```python
from build123d import *

# Parameters (mm, degrees)
SKETCH9_R           = 13.427276503
SKETCH9_R_2         = 5
BOSS_EXTRUDE1_DEPTH = 1
FILLET1_R           = 6
BOSS_EXTRUDE2_START = -3
SKETCH14_R          = 5
BOSS_EXTRUDE2_DEPTH = 5
BOSS_EXTRUDE3_START = -2
SKETCH15_R          = 6
BOSS_EXTRUDE3_DEPTH = 3
CIRPATTERN1_COUNT   = 3


with BuildPart() as part:
    # Sketch9 → Boss-Extrude1 (new body)
    with BuildSketch(Plane.XY):
        with BuildLine():
            Line((-11, 30.049958403), (-11, 21.330729008))
            ThreePointArc((-11, 21.330729008), (-20.784609691, 12), (-23.972953202, -1.139085062))
            Line((-23.972953202, -1.139085062), (-31.524027359, -5.49869976))
            ThreePointArc((-31.524027359, -5.49869976), (-27.712812921, -16), (-20.524027359, -24.551258643))
            Line((-20.524027359, -24.551258643), (-12.972953202, -20.191643945))
            ThreePointArc((-12.972953202, -20.191643945), (0, -24), (12.972953202, -20.191643945))
            Line((12.972953202, -20.191643945), (20.524027359, -24.551258643))
            ThreePointArc((20.524027359, -24.551258643), (27.712812921, -16), (31.524027359, -5.49869976))
            Line((31.524027359, -5.49869976), (23.972953202, -1.139085062))
            ThreePointArc((23.972953202, -1.139085062), (20.784609691, 12), (11, 21.330729008))
            Line((11, 21.330729008), (11, 30.049958403))
            ThreePointArc((11, 30.049958403), (0, 32), (-11, 30.049958403))
        make_face()
        Circle(SKETCH9_R, mode=Mode.SUBTRACT)
        with Locations((0, 24)):
            Circle(SKETCH9_R_2, mode=Mode.SUBTRACT)
        with Locations((20.784609691, -12)):
            Circle(SKETCH9_R_2, mode=Mode.SUBTRACT)
        with Locations((-20.784609691, -12)):
            Circle(SKETCH9_R_2, mode=Mode.SUBTRACT)
    extrude(amount=BOSS_EXTRUDE1_DEPTH)

    # Fillet1
    fillet1_edges = [part.edges().sort_by_distance(p)[0] for p in [
        (11, 30.049958403, 0.5),
        (11, 21.330729008, 0.5),
        (23.972953202, -1.139085062, 0.5),
        (31.524027359, -5.49869976, 0.5),
        (20.524027359, -24.551258643, 0.5),
        (12.972953202, -20.191643945, 0.5),
        (-12.972953202, -20.191643945, 0.5),
        (-20.524027359, -24.551258643, 0.5),
        (-31.524027359, -5.49869976, 0.5),
        (-23.972953202, -1.139085062, 0.5),
        (-11, 21.330729008, 0.5),
        (-11, 30.049958403, 0.5),
    ]]
    fillet(fillet1_edges, radius=FILLET1_R)

    # Sketch14 → Boss-Extrude2 (add)
    with BuildSketch(Plane.XY.offset(1).offset(BOSS_EXTRUDE2_START)):
        with Locations((0, 24)):
            Circle(SKETCH14_R)
    boss_extrude2 = extrude(amount=BOSS_EXTRUDE2_DEPTH)

    # Sketch15 → Boss-Extrude3 (add)
    with BuildSketch(Plane.XY.offset(1).offset(BOSS_EXTRUDE3_START)):
        with Locations((0, 24)):
            Circle(SKETCH15_R)
    boss_extrude3 = extrude(amount=BOSS_EXTRUDE3_DEPTH)

    # CirPattern1: Boss-Extrude2, Boss-Extrude3 ×3 about axis
    cirpattern1_axis = Axis((0, 0, 0), (0, 0, 1))
    add([boss_extrude2.rotate(cirpattern1_axis, i * 360 / CIRPATTERN1_COUNT) for i in range(1, CIRPATTERN1_COUNT)])
    add([boss_extrude3.rotate(cirpattern1_axis, i * 360 / CIRPATTERN1_COUNT) for i in range(1, CIRPATTERN1_COUNT)])


solid = part.part
```
Input: part model. Units: mm. Frame: model coordinates. A direction names the side the tool comes from. Give positions to 0.01 mm unless a question says otherwise; leave off trailing zeros. Order: outer loops, then holes, each group sorted by start corner. A loop starts at its lowest first (then second) coordinate and runs counter-clockwise, first axis right, second up. Notation, with made-up numbers: (34.25, -19) - (78.25, -19) arc R19 ccw to (78.25, 0) - close; hole circle Ø6 at (0, 7.25). An arc over 180 degrees is marked (long way). Put each result on its own line as item: value.
Item 1: Section query B-B, the plane y = 8. Return loops of the section in (x, z), then the cut area to 3 significant figures.
Found:
outline: (-22.63, 0) - (-10.78, 0) - (-10.78, 1) - (-22.63, 1) - close; (10.78, 0) - (22.63, 0) - (22.63, 1) - (10.78, 1) - close
area: 23.7 mm^2
Item 2: Section query D-D, the plane x = 22. Return loops of the section in (y, z), then the cut area to 3 significant figures.
Found:
outline: (-22.58, 0) - (-17.88, 0) - (-17.88, -1) - (-16.85, -1) - (-16.85, -2) - (-7.15, -2) - (-7.15, -1) - (-6.12, -1) - (-6.12, 0) - (9.59, 0) - (9.59, 1) - (-6.12, 1) - (-6.12, 2) - (-7.15, 2) - (-7.15, 3) - (-16.85, 3) - (-16.85, 2) - (-17.88, 2) - (-17.88, 1) - (-22.58, 1) - close
area: 75.1 mm^2
Item 3: Contact query for flat-ended pins moving along their axis: pin 1 (24 mm diameter, centred on x = 0, y = 0, fed in from +Z); pin 2 (0.9 mm diameter, centred on y = 25, z = 0.5, fed in from +X); pin 3 (10 mm diameter, centred on x = 5, y = -17, fed in from -Z); pin 4 (17 mm diameter, centred on x = -8.5, y = 4, fed in from +Z). Output: stop coordinate, or through.
Found:
pin 1: passes through
pin 2: stops at x = 11
pin 3: stops at z = 0
pin 4: stops at z = 1
Item 4: Access query for faces 1 (the cylindrical face through (-2.91, -13.11, 0.49)), 2 (the cylindrical face through (-17.56, -6.94, -0.51)), 3 (the cylindrical face through (-1.301, 18.143, 1.493)). Directions: +Z, -Z, +X, -X, +Y, -Y. A direction counts if a zero-diameter tool reaches every point of the face in a straight line with its end or side. Return the directions, or none.
Found:
face 1: +Z, -Z
face 2: -Z
face 3: +Z
Item 5: Section query C-C, the plane y = 0. Return loops of the section in (x, z), then the cut area to 3 significant figures.
Found:
outline: (-24.39, 0) - (-13.43, 0) - (-13.43, 1) - (-24.39, 1) - close; (13.43, 0) - (24.39, 0) - (24.39, 1) - (13.43, 1) - close
area: 21.9 mm^2
Item 6: Section query A-A, the plane x = 0. Return loops of the section in (y, z).
Found:
outline: (-24, 0) - (-13.43, 0) - (-13.43, 1) - (-24, 1) - close; (13.43, 0) - (18, 0) - (18, -1) - (19, -1) - (19, -2) - (29, -2) - (29, -1) - (30, -1) - (30, 0) - (32, 0) - (32, 1) - (30, 1) - (30, 2) - (29, 2) - (29, 3) - (19, 3) - (19, 2) - (18, 2) - (18, 1) - (13.43, 1) - close
Item 7: Draft query along X for faces 4 (the flat face through (0, 24, 3)), 5 (the cylindrical face through (-30.194, -6.268, 0.507)), 6 (the cylindrical face through (16.362, -7.945, 1.493)), 7 (the cylindrical face through (9.6, 29.37, 0.51)). Return one class per face: +X half, -X half, draft (parallel to the pull), parting line (faces both ways), or undercut.
Found:
face 4: draft
face 5: -X half
face 6: undercut
face 7: +X half
Item 8: Ray query, L1, parallel to X at y = 10, z = 0.8; L2, parallel to Z at x = 15.5, y = -19; L3, parallel to Z at x = 3.5, y = 28. Return the intervals inside material, ascending. Write a range as from..to.
Found:
L1: x = -21.82..-8.96, 8.96..21.82
L2: z = 0..1
L3: z = -1..2
